The listing builds one solid part. Answer for the finished solid, in the listing's coordinates (mm). A direction names the side the tool comes from. Round coordinates to 2 decimals unless told otherwise and drop trailing zeros. Order: outer loops, then holes, each group sorted by start corner. A loop starts at its lowest first (then second) coordinate and runs counter-clockwise, first axis right, second up. Notation, with made-up numbers: (31, -31) -> (51, -31) arc R19 ccw to (51, -9) -> close; hole circle Ø4 at (45, 20.5). An arc over 180 degrees is marked (long way). Return JSON: item names as keys, results as strings. Group by question number.
(1) Each of these flat-tipped pins is pushed along its axis until it touches: pin 1 (8.5 mm diameter, centred on x = -10.2, z = -10.2, fed in from +Y); pin 2 (4 mm diameter, centred on x = -10.2, z = -10.2, fed in from +Y). Where does it stop, or does it pass through?
(2) Consider line 1 (X direction, y = 1.8, z = 10.2); line 2 (X direction, y = 1.15, z = 10.2); line 3 (Z direction, x = 10.2, y = 1.1). Determine where each line is inside the solid, lowest interval first. Write a range as [from, to].
(3) Determine the mould class of faces 3 (the face through (-7.1, 2.7, -13.6)), 4 (the face through (19.1, 2.14, -0.28)), 5 (the face through (8, 2.4, 9)), 6 (the face through (-19.14, 2.1, -0.28)) for opening direction X: +X half, -X half, draft (parallel to the pull), parting line (faces both ways), or undercut.
(4) The part is cut by section D-D (y = 1.6). Determine the outline of the cut face in (x, z), plus the area to 3 significant figures.
(5) Which of the six approach directions +Z, -Z, +X, -X, +Y, -Y give full straight-line access (tool end or side, diameter ignored) to faces 1 (the face through (0.28, 2.1, -19.14)), 2 (the face through (-9, 2.4, -8))?
from build123d import *

# Parameters (mm, degrees)
SKETCH1_W           = 40
SKETCH1_H           = 40
BOSS_EXTRUDE1_DEPTH = 3
SKETCH2_R           = 2.2
CUT_EXTRUDE1_DEPTH  = 29.442925307
SKETCH3_R           = 4.6
CUT_EXTRUDE2_DEPTH  = 0.6
FILLET1_R           = 3


with BuildPart() as part:
    # Sketch1 → Boss-Extrude1 (new body)
    with BuildSketch(Plane(origin=(0, 0, 0), x_dir=(1, 0, 0), z_dir=(0, 1, 0))):
        Rectangle(SKETCH1_W, SKETCH1_H)
    extrude(amount=BOSS_EXTRUDE1_DEPTH)

    # Sketch2 → Cut-Extrude1 (cut, through all)
    with BuildSketch(Plane(origin=(0, 3, 0), x_dir=(1, 0, 0), z_dir=(0, 1, 0))):
        with Locations(Location((-10.2, 10.2, 0), (0, 0, 270))):
            Circle(SKETCH2_R)
        with Locations(Location((10.2, -10.2, 0), (0, 0, 90))):
            Circle(SKETCH2_R)
    extrude(amount=-CUT_EXTRUDE1_DEPTH, mode=Mode.SUBTRACT)

    # Sketch3 → Cut-Extrude2 (cut)
    with BuildSketch(Plane(origin=(0, 3, 0), x_dir=(1, 0, 0), z_dir=(0, 1, 0))):
        with Locations(Location((-10.2, 10.2, 0), (0, 0, 270))):
            Circle(SKETCH3_R)
        with Locations(Location((10.2, -10.2, 0), (0, 0, 270))):
            Circle(SKETCH3_R)
    extrude(amount=-CUT_EXTRUDE2_DEPTH, mode=Mode.SUBTRACT)

    # Fillet1
    fillet1_edges = [part.edges().sort_by_distance(p)[0] for p in [
        (20, 3, 0),
        (-20, 3, 0),
        (0, 3, 20),
        (0, 3, -20),
    ]]
    fillet(fillet1_edges, radius=FILLET1_R - 0.0001)  # a hair under: the kernel refuses the full size


solid = part.part
Answer below:
{
 "1": {"pin 1": "stops at y = 2.4", "pin 2": "passes through"},
 "2": {"line 1": "x = [-19.4, 8], [12.4, 19.4]", "line 2": "x = [-19.77, 8], [12.4, 19.77]", "line 3": "z = [-19.79, 8], [12.4, 19.79]"},
 "3": {"face 3": "undercut", "face 4": "+X half", "face 5": "undercut", "face 6": "-X half"},
 "4": {"outline": "(-19.54, -19.54) -> (19.54, -19.54) -> (19.54, 19.54) -> (-19.54, 19.54) -> close; hole circle Ø4.4 at (-10.2, -10.2); hole circle Ø4.4 at (10.2, 10.2)", "area": "1,500 mm²"},
 "5": {"face 1": "-Z, +X, -X, +Y", "face 2": "+Y"}
}
